Part model, mm, in its own coordinate system. A direction names the side the tool comes from. Give positions to 0.01 mm unless a question says otherwise; leave off trailing zeros. Loops run counter-clockwise (first coordinate to the right, second up) from the corner with the lowest first, then second, coordinate; pieces in that order, holes last. Notation, with made-up numbers: M 2.25,-9 L 47.25,-9 A23 cw 47.25,27 Z; hole C -38,11.5 d8. An arc over 180 degrees is marked long. Put each result on its own line as item: value. Start each with the question number.
```python
from build123d import *

# Parameters (mm, degrees)
BOSS_EXTRUDE1_DEPTH             = 20
TAP_DRILL_FOR_M4X0_7_TAP1_D     = 3.3
TAP_DRILL_FOR_M4X0_7_TAP1_DEPTH = 5
TAP_DRILL_FOR_M4X0_7_TAP1_TIP   = 0.991420021
TAP_DRILL_FOR_M5X0_8_TAP3_D     = 4.2
TAP_DRILL_FOR_M5X0_8_TAP2_D     = 4.2
TAP_DRILL_FOR_M5X0_8_TAP2_DEPTH = 7
TAP_DRILL_FOR_M5X0_8_TAP2_TIP   = 1.2618073
FILLET1_R                       = 1


with BuildPart() as part:
    # Sketch1 → Boss-Extrude1 (new body)
    with BuildSketch(Plane.XY):
        Polygon((22.5, 40), (-80, 40), (-80, 0), (80, 0), (80, 40), (57.5, 40), (57.5, 23), (57.5, 22.95), (43, 22.95), (43, 17), (37, 17), (37, 22.95), (22.5, 22.95), (22.5, 23), align=None)
    extrude(amount=-BOSS_EXTRUDE1_DEPTH)

    # Tap Drill for M4x0.7 Tap1
    with Locations(Plane(origin=(30, 22.95, -4), x_dir=(0, 0, 1), z_dir=(0, 1, 0))):
        with Locations((0, 0), (0, 20), (-12, 0), (-12, 20)):
            Hole(TAP_DRILL_FOR_M4X0_7_TAP1_D / 2, depth=TAP_DRILL_FOR_M4X0_7_TAP1_DEPTH)
            with Locations((0, 0, -(TAP_DRILL_FOR_M4X0_7_TAP1_DEPTH + TAP_DRILL_FOR_M4X0_7_TAP1_TIP / 2))):  # 118° drill point
                Cone(0, TAP_DRILL_FOR_M4X0_7_TAP1_D / 2, TAP_DRILL_FOR_M4X0_7_TAP1_TIP, mode=Mode.SUBTRACT)

    # Tap Drill for M5x0.8 Tap3 (through all)
    with Locations(Plane(origin=(-70, 30, 0), x_dir=(1, 0, 0), z_dir=(0, 0, 1))):
        with Locations((0, 0), (0, -20), (140, -20), (140, 0)):
            Hole(TAP_DRILL_FOR_M5X0_8_TAP3_D / 2)

    # Tap Drill for M5x0.8 Tap2
    with Locations(Plane(origin=(-60, 0, -10), x_dir=(-1, 0, 0), z_dir=(0, -1, 0))):
        with Locations((0, 0), (-60, 0), (-120, 0)):
            Hole(TAP_DRILL_FOR_M5X0_8_TAP2_D / 2, depth=TAP_DRILL_FOR_M5X0_8_TAP2_DEPTH)
            with Locations((0, 0, -(TAP_DRILL_FOR_M5X0_8_TAP2_DEPTH + TAP_DRILL_FOR_M5X0_8_TAP2_TIP / 2))):  # 118° drill point
                Cone(0, TAP_DRILL_FOR_M5X0_8_TAP2_D / 2, TAP_DRILL_FOR_M5X0_8_TAP2_TIP, mode=Mode.SUBTRACT)

    # Fillet1
    fillet1_edges = [part.edges().sort_by_distance(p)[0] for p in [
        (57.5, 40, -10),
        (22.5, 40, -10),
    ]]
    fillet(fillet1_edges, radius=FILLET1_R)


solid = part.part
```
1) Wall check: L1, parallel to X at y = 5.25, z = -10; L2, parallel to Y at x = -70, z = -7.25; L3, parallel to Z at x = 60, y = 2. Give the ranges that are in metal, low to high.
2) Which spindle directions (+Z, -Z, +X, -X, +Y, -Y) get a long thin tool onto all of the face, cutting with end or side? Do faces 4 (the cylindrical face through (-0.273, 3.549, -12.082)), 5 (the cylindrical face through (51.39, 20.42, -16.89)), 6 (the flat face through (50, 22.95, -10)). Say none if no direction does.
3) Mould opens along Y. For faces 1 (the flat face through (69, 40, -10)), 2 (the cylindrical face through (70.46, 27.95, -10.14)), 3 (the flat face through (22.5, 31, -10)) say: +Y half, -Y half, draft (parallel to the pull), parting line (faces both ways), or undercut.
4) Band-saw the part on A-A on y = 26. Give the cut face in (x, z), then the cut area to 3 significant figures.
5) Band-saw the part on B-B on y = 10. Give the cut face in (x, z).
6) Pin check, flat tips, straight feed: pin 1 Ø6.5 at (x, y) = (70, 30) entering from -Z; pin 2 Ø11.5 at (x, z) = (49.5, -5) entering from +Y; pin 3 Ø3.5 at (x, z) = (0, -10) entering from -Y; pin 4 Ø4 at (x, y) = (70, 10) entering from -Z. Stop position of each tip, or through.
Evaluation:
1. L1: -80 to -62.1, -57.9 to -2.1, 2.1 to 57.9, 62.1 to 80
1. L2: 0 to 7.9, 12.1 to 27.9, 32.1 to 40
1. L3: -20 to -12.1, -7.9 to 0
2. face 4: -Y
2. face 5: +Y
2. face 6: +Z, -Z, +Y
3. face 1: +Y half
3. face 2: undercut
3. face 3: draft
4. outline: M -80,-20 L 22.5,-20 L 22.5,0 L -80,0 Z; M 57.5,-20 L 80,-20 L 80,0 L 57.5,0 Z
4. area: 2,500 mm2
5. outline: M -80,-20 L -72.1,-20 L -72.1,0 L -80,0 Z; M -67.9,-20 L 67.9,-20 L 67.9,0 L -67.9,0 Z; M 72.1,-20 L 80,-20 L 80,0 L 72.1,0 Z
6. pin 1: z = -20
6. pin 2: y = 22.95
6. pin 3: y = 7.21
6. pin 4: through
